Source: CAD feature listing. Evaluate the final solid. Frame: model axes, mm. Face numbers are marked on the shaded views. A direction names the side the tool comes from. Round coordinates to 2 decimals unless told otherwise and drop trailing zeros. Loops run counter-clockwise (first coordinate to the right, second up) from the corner with the lowest first, then second, coordinate; pieces in that order, holes last. Notation, with made-up numbers: (88.5, 53) - (134.5, 53) arc R18 ccw to (134.5, 67) - close; hole circle Ø8 at (24.25, -2.5). An arc over 180 degrees is marked (long way). Write item = value, one per line. Start each with the question number.
from build123d import *

# Parameters (mm, degrees)
SKETCH1_W           = 200
SKETCH1_H           = 200
BOSS_EXTRUDE1_DEPTH = 140
SHELL2_T            = 10
CUT_EXTRUDE2_DEPTH  = 264.818119165
CUT_EXTRUDE3_DEPTH  = 264.818119165
SKETCH4_W           = 180
SKETCH4_H           = 180
BOSS_EXTRUDE3_DEPTH = 4


with BuildPart() as part:
    # Sketch1 → Boss-Extrude1 (new body)
    with BuildSketch(Plane(origin=(0, 0, 0), x_dir=(1, 0, 0), z_dir=(0, 1, 0))):
        Rectangle(SKETCH1_W, SKETCH1_H)
    extrude(amount=BOSS_EXTRUDE1_DEPTH)

    # Shell2 (no face opened: a closed hollow body)
    add(offset(amount=-SHELL2_T, mode=Mode.PRIVATE), mode=Mode.SUBTRACT)

    # Sketch2 → Cut-Extrude2 (cut, through all)
    with BuildSketch(Plane(origin=(100, 0, 0), x_dir=(0, 0, -1), z_dir=(1, 0, 0))):
        Polygon((-30, 40), (-4, 40), (-4, 10), (-90, 10), (-90, 66), (-30, 66), align=None)
        Polygon((-30, 100), (-4, 100), (-4, 130), (-90, 130), (-90, 74), (-30, 74), align=None)
        Polygon((30, 40), (30, 66), (90, 66), (90, 10), (4, 10), (4, 40), align=None)
        Polygon((30, 74), (30, 100), (4, 100), (4, 130), (90, 130), (90, 74), align=None)
    extrude(amount=-CUT_EXTRUDE2_DEPTH, mode=Mode.SUBTRACT)

    # Sketch3 → Cut-Extrude3 (cut, through all)
    with BuildSketch(Plane.XY.offset(100)):
        Polygon((3.383720977, 39.438488697), (3.383720977, 10), (90, 10), (90, 65.438488697), (29.383720977, 65.438488697), (29.383720977, 39.438488697), align=None)
        Polygon((3.383720977, 130), (90, 130), (90, 73.438488697), (29.383720977, 73.438488697), (29.383720977, 99.438488697), (3.383720977, 99.438488697), align=None)
        Polygon((-90, 130), (-4.616279023, 130), (-4.616279023, 99.438488697), (-30.616279023, 99.438488697), (-30.616279023, 73.438488697), (-90, 73.438488697), align=None)
        Polygon((-30.616279023, 65.438488697), (-90, 65.438488697), (-90, 10), (-4.616279023, 10), (-4.616279023, 39.438488697), (-30.616279023, 39.438488697), align=None)
    extrude(amount=-CUT_EXTRUDE3_DEPTH, mode=Mode.SUBTRACT)

    # Sketch4 → Boss-Extrude3 (add)
    with BuildSketch(Plane(origin=(29.307172117, 70, -14.72040922), x_dir=(1, 0, 0), z_dir=(0, 1, 0))):
        with Locations((-29.307172117, -14.72040922)):
            Rectangle(SKETCH4_W, SKETCH4_H)
    extrude(amount=-BOSS_EXTRUDE3_DEPTH)


solid = part.part
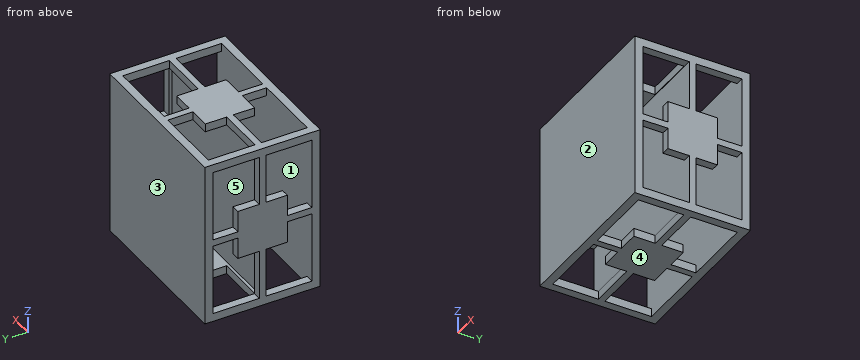
(1) Mould query, pull axis Y, two halves, no side actions, for the marked faces 3, 4 and 5. Classes: +Y half, -Y half, draft (parallel to the pull), parting line (faces both ways), or undercut.
(2) Access query for the marked faces 1 and 2. Directions: +Z, -Z, +X, -X, +Y, -Y. A direction counts if a zero-diameter tool reaches every point of the face in a straight line with its end or side. Return the directions, or none.
(3) Material intervals for line 1 along Y through (x, z) = (17, -37.5); line 2 along Z through (x, y) = (3, 34.5), sorted ascending. Write a range as from..to.
(4) Cut plane A-A (y = 126.5). State how many separate pieces and enclosed holes the cut face has, and give its area (3 significant figures).
(5) Cut plane C-C (x = 65). Output: boundary loops of the cut face in (y, z).
(6) Pin query (flat end, axial travel): P1, Ø5, axis at x = -24.5, z = -50.5, coming from the -Y side. Return the tip coordinate at first contact, or that it passes through.
(7) Cut plane B-B (z = 54.5). Output: boundary loops of the cut face in (x, y), and give its area (3 significant figures).
Solution:
q1.face_3 = +Y half
q1.face_4 = draft
q1.face_5 = undercut
q2.face_1 = none
q2.face_2 = +Z, -Z, +X, -X, -Y
q3.line_1 = 0..10, 66..70, 130..140
q3.line_2 = -100..-90, 90..100
q4.separate_pieces = 8
q4.enclosed_holes = 0
q4.area = 720 mm^2
q5.outline = (0, -100) - (10, -100) - (10, 100) - (0, 100) - close; (65.44, -100) - (73.44, -100) - (73.44, -90) - (70, -90) - (70, 90) - (73.44, 90) - (73.44, 100) - (65.44, 100) - (65.44, 90) - (66, 90) - (66, -90) - (65.44, -90) - close; (130, -100) - (140, -100) - (140, 100) - (130, 100) - close
q6.P1 = 0
q7.outline = (-100, 0) - (100, 0) - (100, 10) - (-100, 10) - close; (-100, 66) - (100, 66) - (100, 74) - (90, 74) - (90, 70) - (-90, 70) - (-90, 74) - (-100, 74) - close; (-100, 130) - (100, 130) - (100, 140) - (-100, 140) - close
q7.area = 4,880 mm^2
